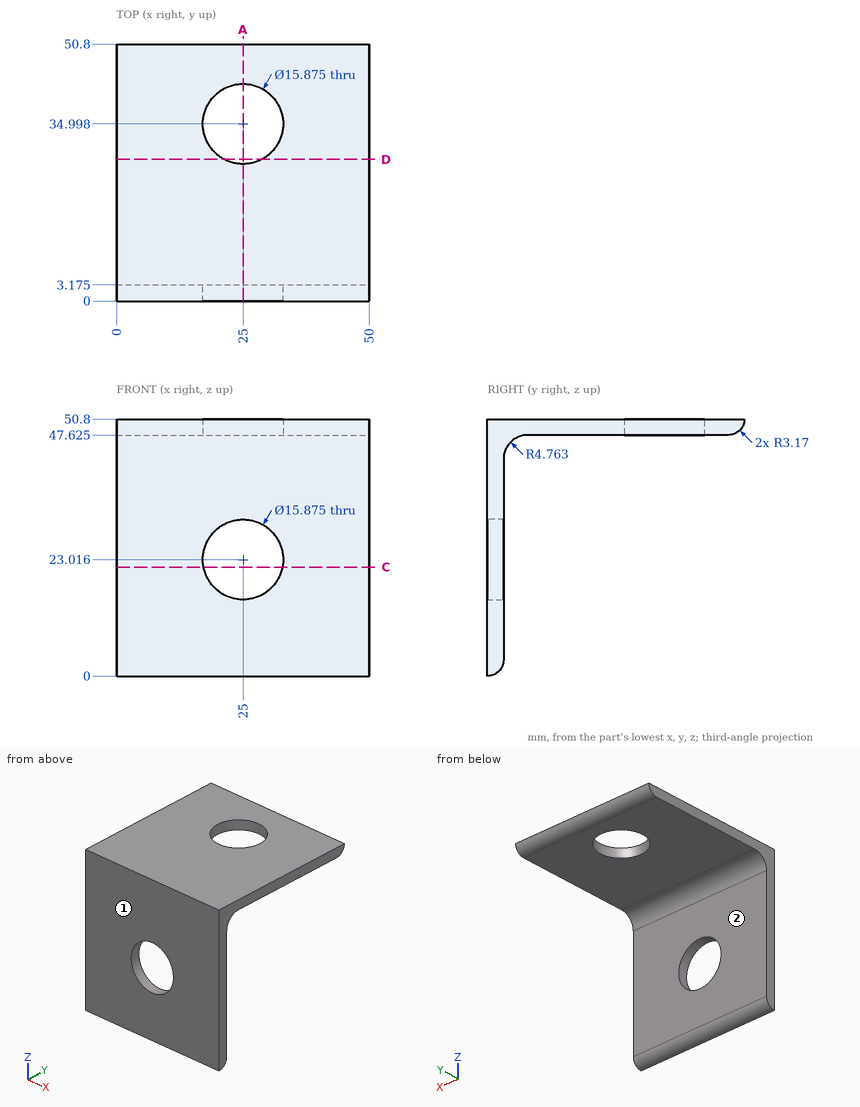
The figure shows three views and two pictorial views of one solid part (mm, origin at its lowest corner). Answer the questions. A direction names the side the tool comes from. Round coordinates to 2 decimals unless told otherwise and drop trailing zeros. Order: outer loops, then holes, each group sorted by start corner. A loop starts at its lowest first (then second) coordinate and runs counter-clockwise, first axis right, second up. Notation, with made-up numbers: (-39, 39) - (-7, 39) arc R20 ccw to (-7, 71) - close; hole circle Ø4 at (76.5, 87). An arc over 180 degrees is marked (long way). Write item = value, one per line. Start each with the question number.
1) Straight lines are drawn through the part: L1, parallel to Y at x = 34, z = 40.5 (1 decimal); L2, parallel to Z at x = 43, y = 24.5 (1 decimal); L3, parallel to Y at x = 3, z = 48 (1 decimal). For each, find the intervals that lie inside material, in ascending order.
2) Section A-A, the plane x = 25 is taken. Count the separate pieces of the cut face and the enclosed holes in it, plus the area to 3 significant figures.
3) For the marked faces 1 and 2, determine the directions among +Z, -Z, +X, -X, +Y, -Y from which every point of the face is accessible in a straight line to the end or side of a thin tool.
4) Given pin 1 (12 mm diameter, centred on x = 24.5, y = 26, fed in from -Z) (1 decimal); pin 2 (5 mm diameter, centred on x = 35, z = 12, fed in from +Y) (1 decimal); pin 3 (9.5 mm diameter, centred on x = 25, z = 23.02, fed in from +Y), each flat-ended and moving along its own axis, determine where each tip first touches the part or whether it passes through.
5) Section C-C, the plane z = 21.5 is taken. Write down the section's boundary in (x, y) (1 decimal).
6) Section D-D, the plane y = 28 is taken. Write down the section's boundary in (x, z) (1 decimal).
Results list:
q1.L1 = 0 to 3.2
q1.L2 = 47.6 to 50.8
q1.L3 = 0 to 49.1
q2.separate_pieces = 3
q2.enclosed_holes = 0
q2.area = 212 mm^2
q3.face_1 = +Z, -Z, +X, -X, -Y
q3.face_2 = -Z, +X, -X, +Y
q4.pin_1 = 47.6
q4.pin_2 = 3.2
q4.pin_3 = through
q5.outline = (0, 0) - (17.2, 0) - (17.2, 3.2) - (0, 3.2) - close; (32.8, 0) - (50, 0) - (50, 3.2) - (32.8, 3.2) - close
q6.outline = (0, 47.6) - (21.3, 47.6) - (21.3, 50.8) - (0, 50.8) - close; (28.7, 47.6) - (50, 47.6) - (50, 50.8) - (28.7, 50.8) - close
